Input: part model. Units: mm. Frame: model coordinates. A direction names the side the tool comes from. Give positions to 0.01 mm unless a question says otherwise; leave off trailing zeros. Loops run counter-clockwise (first coordinate to the right, second up) from the corner with the lowest first, then second, coordinate; pieces in that order, holes last. Notation, with made-up numbers: (50, 19) -> (104, 19) arc R19 ccw to (104, 56) -> close; hole circle Ø5 at (54, -17.75). An arc over 180 degrees is marked (long way). One line per question, with ' | ' between items.
from build123d import *

# Parameters (mm, degrees)
SKETCH1_R           = 24
BOSS_EXTRUDE1_DEPTH = 6
SKETCH2_R           = 2
CUT_EXTRUDE1_DEPTH  = 2
SKETCH3_R           = 1.25
CUT_EXTRUDE2_DEPTH  = 35.176014981
SKETCH4_R           = 12.5
BOSS_EXTRUDE2_DEPTH = 60
SKETCH5_R           = 8.5
CUT_EXTRUDE3_DEPTH  = 5
FILLET1_R           = 1
SKETCH6_R           = 2
CUT_EXTRUDE4_DEPTH  = 20


with BuildPart() as part:
    # Sketch1 → Boss-Extrude1 (new body)
    with BuildSketch(Plane(origin=(0, 0, 0), x_dir=(1, 0, 0), z_dir=(0, 1, 0))):
        with Locations(Location((0, 0, 0), (0, 0, 270))):
            Circle(SKETCH1_R)
    extrude(amount=BOSS_EXTRUDE1_DEPTH)

    # Sketch2 → Cut-Extrude1 (cut)
    with BuildSketch(Plane(origin=(0, 6, 0), x_dir=(1, 0, 0), z_dir=(0, 1, 0))):
        with Locations(Location((0, 18, 0), (0, 0, 270))):
            Circle(SKETCH2_R)
        with Locations(Location((9, 15.588457268, 0), (0, 0, 270))):
            Circle(SKETCH2_R)
        with Locations(Location((15.588457268, 9, 0), (0, 0, 270))):
            Circle(SKETCH2_R)
        with Locations(Location((18, 0, 0), (0, 0, 270))):
            Circle(SKETCH2_R)
        with Locations(Location((15.588457268, -9, 0), (0, 0, 270))):
            Circle(SKETCH2_R)
        with Locations(Location((9, -15.588457268, 0), (0, 0, 270))):
            Circle(SKETCH2_R)
        with Locations(Location((0, -18, 0), (0, 0, 270))):
            Circle(SKETCH2_R)
        with Locations(Location((-9, -15.588457268, 0), (0, 0, 270))):
            Circle(SKETCH2_R)
        with Locations(Location((-15.588457268, -9, 0), (0, 0, 270))):
            Circle(SKETCH2_R)
        with Locations(Location((-18, 0, 0), (0, 0, 270))):
            Circle(SKETCH2_R)
        with Locations(Location((-15.588457268, 9, 0), (0, 0, 270))):
            Circle(SKETCH2_R)
        with Locations(Location((-9, 15.588457268, 0), (0, 0, 270))):
            Circle(SKETCH2_R)
    extrude(amount=-CUT_EXTRUDE1_DEPTH, mode=Mode.SUBTRACT)

    # Sketch3 → Cut-Extrude2 (cut, through all)
    with BuildSketch(Plane(origin=(0, 4, 0), x_dir=(1, 0, 0), z_dir=(0, 1, 0))):
        with Locations(Location((0, 18, 0), (0, 0, 270))):
            Circle(SKETCH3_R)
        with Locations(Location((9, 15.588457268, 0), (0, 0, 270))):
            Circle(SKETCH3_R)
        with Locations(Location((15.588457268, 9, 0), (0, 0, 270))):
            Circle(SKETCH3_R)
        with Locations(Location((18, 0, 0), (0, 0, 270))):
            Circle(SKETCH3_R)
        with Locations(Location((15.588457268, -9, 0), (0, 0, 270))):
            Circle(SKETCH3_R)
        with Locations(Location((9, -15.588457268, 0), (0, 0, 270))):
            Circle(SKETCH3_R)
        with Locations(Location((0, -18, 0), (0, 0, 270))):
            Circle(SKETCH3_R)
        with Locations(Location((-9, -15.588457268, 0), (0, 0, 270))):
            Circle(SKETCH3_R)
        with Locations(Location((-15.588457268, -9, 0), (0, 0, 270))):
            Circle(SKETCH3_R)
        with Locations(Location((-18, 0, 0), (0, 0, 270))):
            Circle(SKETCH3_R)
        with Locations(Location((-15.588457268, 9, 0), (0, 0, 270))):
            Circle(SKETCH3_R)
        with Locations(Location((-9, 15.588457268, 0), (0, 0, 270))):
            Circle(SKETCH3_R)
    extrude(amount=-CUT_EXTRUDE2_DEPTH, mode=Mode.SUBTRACT)

    # Sketch4 → Boss-Extrude2 (add)
    with BuildSketch(Plane(origin=(0, 6, 0), x_dir=(1, 0, 0), z_dir=(0, 1, 0))):
        with Locations(Location((0, 0, 0), (0, 0, 270))):
            Circle(SKETCH4_R)
    extrude(amount=BOSS_EXTRUDE2_DEPTH)

    # Sketch5 → Cut-Extrude3 (cut)
    with BuildSketch(Plane.XZ):
        with Locations(Location((0, 0, 0), (0, 0, 270))):
            Circle(SKETCH5_R)
    extrude(amount=-CUT_EXTRUDE3_DEPTH, mode=Mode.SUBTRACT)

    # Fillet1
    fillet1_edges = [part.edges().sort_by_distance(p)[0] for p in [
        (0, 6, -24),
    ]]
    fillet(fillet1_edges, radius=FILLET1_R)

    # Sketch6 → Cut-Extrude4 (cut)
    with BuildSketch(Plane(origin=(0, 66, 0), x_dir=(1, 0, 0), z_dir=(0, 1, 0))):
        with Locations(Location((0, 8, 0), (0, 0, 270))):
            Circle(SKETCH6_R)
        with Locations(Location((8, 0, 0), (0, 0, 270))):
            Circle(SKETCH6_R)
        with Locations(Location((0, -8, 0), (0, 0, 270))):
            Circle(SKETCH6_R)
        with Locations(Location((-8, 0, 0), (0, 0, 270))):
            Circle(SKETCH6_R)
    extrude(amount=-CUT_EXTRUDE4_DEPTH, mode=Mode.SUBTRACT)


solid = part.part
1. Pull-direction query (X, two-part tool) for faces 4 (the cylindrical face through (7.21, 2.46, 22.89)), 5 (the flat face through (17, 4, 10)), 6 (the cylindrical face through (8.428, 2.465, 1.107)); classes: pulls with the +X half, pulls with the -X half, needs draft (parallel to the pull), parting line crosses it, or undercut.
Determined:
face 4: parting line crosses it | face 5: undercut | face 6: undercut
2. Section query B-B (z = 0). Count the separate pieces of the cut face and the enclosed holes in it, then the cut area to 3 significant figures.
Determined:
separate pieces: 3 | enclosed holes: 0 | area: 1,510 mm2
3. Section query A-A (y = 52.5). Output: boundary loops of the cut face in (x, z), then the cut area to 3 significant figures.
Determined:
outline: circle Ø25 at (0, 0); hole circle Ø4 at (-8, 0); hole circle Ø4 at (0, -8); hole circle Ø4 at (0, 8); hole circle Ø4 at (8, 0) | area: 441 mm2
4. Pin query (flat end, axial travel): P1, Ø3, axis at y = 24, z = 6, coming from the +X side; P2, Ø10, axis at x = -8, y = 20.5, coming from the +Z side; P3, Ø4, axis at x = 18, z = 0, coming from the -Y side; P4, Ø3, axis at x = -15.5, z = -9, coming from the +Y side. Return the tip coordinate at first contact, or that it passes through.
Determined:
P1: stops at x = 11.66 | P2: stops at z = 12.13 | P3: stops at y = 0 | P4: stops at y = 4
5. Ray query, line 1 along Y through (x, z) = (-13, -12.5); line 2 along Y through (x, z) = (-1, 0); line 3 along X through (y, z) = (3, 9). Return the intervals inside material, ascending. Write a range as from..to.
Determined:
line 1: y = 0..6 | line 2: y = 5..66 | line 3: x = -22.25..-16.84, -14.34..14.34, 16.84..22.25
6. Section query C-C (y = 28.5). Output: boundary loops of the cut face in (x, z), then the cut area to 3 significant figures.
Determined:
outline: circle Ø25 at (0, 0) | area: 491 mm2
7. Reachability of faces 1 (the flat face through (0, 5, 0)), 2 (the cylindrical face through (-16.946, 2.028, 0.672)), 3 (the cylindrical face through (10.352, 5.014, -17.063)) from +Z, -Z, +X, -X, +Y, -Y: full face, straight path, thin tool, end or side. Return the list, or none.
Determined:
face 1: -Y | face 2: +Y, -Y | face 3: +Y
